from build123d import *

# Parameters (mm, degrees)
F1_DEPTH  = 5
F3_DEPTH  = 3.1
F4_R      = 2.25
F5_DEPTH  = 5.001
F6_W      = 32
F6_H      = 2.5
F7_DEPTH  = 8.5
F8_W      = 32
F8_H      = 2.75
F9_DEPTH  = 4.5
F10_W     = 32
F10_H     = 2.5
F11_DEPTH = 10.75
F12_R     = 1.35
F13_DEPTH = 3
F14_DEPTH = 2.5


# Not quite as in the source:
# - a feature names something its author has since deleted; it is built from what else it names


with BuildPart() as f1:
    # F0 (on Top) → F1 (new body)
    with BuildSketch(Plane.XY):
        with BuildLine():
            Line((0, 2.5), (0, 0))
            Line((0, 0), (43, 0))
            Line((43, 0), (43, 9))
            ThreePointArc((43, 9), (41.8284271247, 11.8284271247), (39, 13))
            Line((39, 13), (33.8239016482, 13))
            ThreePointArc((33.8239016482, 13), (31.5169659003, 12.2677281794), (30.0546821723, 10.3390237274))
            Line((30.0546821723, 10.3390237274), (29.1077482568, 7.6734983272))
            ThreePointArc((29.1077482568, 7.6734983272), (27.8028764103, 5.8618093159), (25.7302204856, 5.0317460488))
            Line((25.7302204856, 5.0317460488), (0, 2.5))
        make_face()
    extrude(amount=F1_DEPTH)

    # F2 (on face) → F3 (cut)
    with BuildSketch(Plane.XY.offset(5)):
        Polygon((39.9846022951, 8.7502746915), (36.3578632635, 10.7817185123), (32.7852117926, 8.6565922885), (32.8392993532, 4.5000222439), (36.4660383847, 2.4685784231), (40.0386898557, 4.5937046469), align=None)
    extrude(amount=-F3_DEPTH, mode=Mode.SUBTRACT)

    # F4 (on face) → F5 (cut, through all)
    with BuildSketch(Plane(origin=(0, 0, 0), x_dir=(1, 0, 0), z_dir=(0, 0, -1))):
        with Locations((36.4119508241, -6.4989285606)):
            Circle(F4_R)
    extrude(amount=-F5_DEPTH, mode=Mode.SUBTRACT)

    # F6 (on face) → F7 (join)
    with BuildSketch(Plane.XY.offset(5)):
        with Locations((16, 1.25)):
            Rectangle(F6_W, F6_H)
    extrude(amount=F7_DEPTH)

    # F8 (on face) → F9 (join)
    with BuildSketch(Plane.XZ):
        with Locations((16, 12.125)):
            Rectangle(F8_W, F8_H)
    extrude(amount=F9_DEPTH)

    # F10 (on face) → F11 (join)
    with BuildSketch(Plane(origin=(0, 0, 10.75), x_dir=(1, 0, 0), z_dir=(0, 0, -1))):
        with Locations((16, 3.25)):
            Rectangle(F10_W, F10_H)
    extrude(amount=F11_DEPTH)

    # F12 (on face) → F13 (join)
    with BuildSketch(Plane(origin=(0, 2.5, 0), x_dir=(-1, 0, 0), z_dir=(0, 1, 0))):
        with BuildLine():
            Line((-27.1456439237, 5), (-24.8543560763, 5))
            ThreePointArc((-24.8543560763, 5), (-26, 10.25), (-27.1456439237, 5))
        make_face()
        with Locations((-26, 7.5)):
            Circle(F12_R, mode=Mode.SUBTRACT)
        with BuildLine():
            Line((-7.1456439237, 5), (-4.8543560763, 5))
            ThreePointArc((-4.8543560763, 5), (-6, 10.25), (-7.1456439237, 5))
        make_face()
        with Locations((-6, 7.5)):
            Circle(F12_R, mode=Mode.SUBTRACT)
    extrude(amount=F13_DEPTH)

    # F14 (cut, through all): faces of the model
    f14_faces = [f1.faces().sort_by_distance(p)[0] for p in [
        (6, 2.5, 7.5),
        (26, 2.5, 7.5),
    ]]
    extrude(f14_faces, amount=-F14_DEPTH, mode=Mode.SUBTRACT)


solid = f1.part
Can you work these out from the model? Positions are in its coordinate system, mm. A direction names the side the tool comes from. Coordinates: 2 decimals unless noted, no trailing zeros. Loops run counter-clockwise (first coordinate to the right, second up) from the corner with the lowest first, then second, coordinate; pieces in that order, holes last. Notation, with made-up numbers: (41, 12.25) - (78, 12.25) arc R16 cw to (78, 25.25) - close; hole circle Ø11 at (31, -34.75). An arc over 180 degrees is marked (long way). Put each result on its own line as item: value. Start each with the question number.
Item 1: If we mould it in two halves opening along Z, with no side actions, what happens to faces 1 (the face through (34.627, 3.499, 3.472)), 2 (the face through (25.9, 3.98, 10.25)), 3 (the face through (16, -3, 0)), 4 (the face through (34.7, 4.8, 1.9))? For each: +Z half, -Z half, draft (parallel to the pull), parting line (faces both ways), or undercut.
Item 2: Suppose I cut it at D-D (z = 1.5). Please give me the cut outline in (x, y), and give its area (3 significant figures).
Item 3: Suppose I cut it at B-B (z = 7.5). Please give me the cut outline in (x, y), and give its area (3 significant figures).
Item 4: If I drill on line 1 along Y through (x, z) = (31.5, 9.75); line 2 along Z through (x, y) = (26, 3.9); line 3 along X through (y, z) = (0.25, 8.25), over which ranges is the centre line in solid material (lowest first)?
Item 5: Suppose I cut it at C-C (x = 38). Please give me the cut outline in (y, z) (3 decimals), and give its area (3 significant figures).
Item 6: Which directions (+Z, -Z, +X, -X, +Y, -Y) give clear straight access to the entire face, cutting with the end or side of a thin tool? Please do faces 5 (the face through (13.045, 3.784, 2.465)), 6 (the face through (38.2, 3.5, 3.5)), 7 (the face through (16, -4.5, 7)), 8 (the face through (18, 3, 5)).
Item 7: For pin 1 (6 mm diameter, centred on x = 29.5, y = 9, fed in from +Z); pin 2 (2 mm diameter, centred on x = 25.5, y = 4.5, fed in from +Z); pin 3 (3 mm diameter, centred on x = 23.5, z = 3, fed in from +Y), each with a flat end and sliding along its axis, tell me the tip position at first contact or that it passes through.
Item 8: Suppose I cut it at A-A (z = 3.75). Please give me the cut outline in (x, y), and give its area (3 significant figures).
Here are the results:
1. face 1: draft
1. face 2: undercut
1. face 3: -Z half
1. face 4: +Z half
2. outline: (0, -4.5) - (32, -4.5) - (32, -2) - (0, -2) - close; (0, 0) - (43, 0) - (43, 9) arc R4 ccw to (39, 13) - (33.82, 13) arc R4 ccw to (30.05, 10.34) - (29.11, 7.67) arc R4 cw to (25.73, 5.03) - (0, 2.5) - close; hole circle Ø4.5 at (36.41, 6.5)
2. area: 351 mm²
3. outline: (0, -4.5) - (32, -4.5) - (32, -2) - (0, -2) - close; (0, 0) - (4.65, 0) - (4.65, 5.5) - (3.25, 5.5) - (3.25, 2.5) - (0, 2.5) - close; (7.35, 0) - (24.65, 0) - (24.65, 5.5) - (23.25, 5.5) - (23.25, 2.5) - (8.75, 2.5) - (8.75, 5.5) - (7.35, 5.5) - close; (27.35, 0) - (32, 0) - (32, 2.5) - (28.75, 2.5) - (28.75, 5.5) - (27.35, 5.5) - close
3. area: 163 mm²
4. line 1: -4.5 to -2, 0 to 2.5
4. line 2: 0 to 6.15, 8.85 to 10.25
4. line 3: 0 to 4.88, 7.12 to 24.88, 27.12 to 32
5. outline: (0, 0) - (4.905, 0) - (4.905, 1.9) - (3.381, 1.9) - (3.381, 5) - (0, 5) - close; (8.093, 0) - (13, 0) - (13, 5) - (9.862, 5) - (9.862, 1.9) - (8.093, 1.9) - close
5. area: 38.9 mm²
6. face 5: -Z, -X, +Y
6. face 6: +Z
6. face 7: +Z, -Z, +X, -X, -Y
6. face 8: +Y
7. pin 1: z = 5
7. pin 2: z = 10.25
7. pin 3: y = 4.96
8. outline: (0, -4.5) - (32, -4.5) - (32, -2) - (0, -2) - close; (0, 0) - (43, 0) - (43, 9) arc R4 ccw to (39, 13) - (33.82, 13) arc R4 ccw to (30.05, 10.34) - (29.11, 7.67) arc R4 cw to (25.73, 5.03) - (0, 2.5) - close; hole (32.79, 8.66) - (32.84, 4.5) - (36.47, 2.47) - (40.04, 4.59) - (39.98, 8.75) - (36.36, 10.78) - close
8. area: 322 mm²
